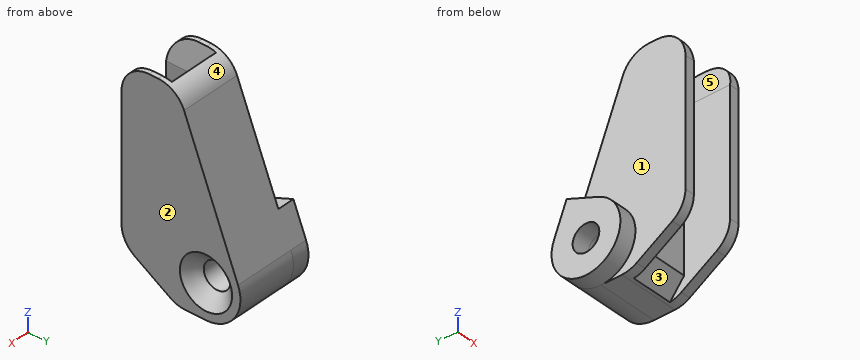
from build123d import *
from OCP.BRepFilletAPI import BRepFilletAPI_MakeChamfer

# Parameters (mm, degrees)
SKETCH1_R                                       = 2.2
BOSS_EXTRUDE1_DEPTH                             = 11
CUT_EXTRUDE1_REACH                              = 42.774
SKETCH2_W                                       = 7.5
SKETCH2_H                                       = 8.25
CHAMFER3_SIZE                                   = 5
CHAMFER3_SIZE2                                  = 0.881634904
FILLET1_R                                       = 5
CHAMFER1_SIZE                                   = 2.212207332
CHAMFER1_SIZE_2                                 = 4
CSK_FOR_M4_FLAT_HEAD_MACHINE_SCREW1_D           = 4.8
CSK_FOR_M4_FLAT_HEAD_MACHINE_SCREW1_CSINK_D     = 9.4
CSK_FOR_M4_FLAT_HEAD_MACHINE_SCREW1_CSINK_ANGLE = 90
BOSS_EXTRUDE2_START                             = 3.12
SKETCH6_R                                       = 2.4
BOSS_EXTRUDE2_DEPTH                             = 3.12


with BuildPart() as part:
    # Sketch1 → Boss-Extrude1 (new body)
    with BuildSketch(Plane(origin=(0, 0, 0), x_dir=(0, 0, -1), z_dir=(1, 0, 0))):
        with BuildLine():
            Line((-30, -15.2), (-30, -5.2))
            Line((-30, -5.2), (-2.280651189, 5.765295322))
            ThreePointArc((-2.280651189, 5.765295322), (3.485682331, 5.12737932), (6.2, 0))
            Line((6.2, 0), (6.2, -5.2))
            Line((6.2, -5.2), (0, -15.2))
            Line((0, -15.2), (-30, -15.2))
        make_face()
        Circle(SKETCH1_R, mode=Mode.SUBTRACT)
    extrude(amount=BOSS_EXTRUDE1_DEPTH)

    # Cut-Extrude1: up to this plane
    cut_extrude1_end = Plane(origin=(11, -5.2, -6.2), z_dir=(0, 0.5269396688616753, 0.8499026917123795))
    # Sketch2 → Cut-Extrude1 (cut, up to the surface)
    with BuildSketch(Plane.XY.offset(30), mode=Mode.PRIVATE) as cut_extrude1_sk1:
        with Locations((5.5, -11.075)):
            Rectangle(SKETCH2_W, SKETCH2_H)
    cut_extrude1_tool1 = split(extrude(cut_extrude1_sk1.sketch, amount=-CUT_EXTRUDE1_REACH, mode=Mode.PRIVATE), bisect_by=cut_extrude1_end, keep=Keep.BOTH, mode=Mode.PRIVATE)
    add(cut_extrude1_tool1.solids().sort_by_distance((5.5, -11.075, 30))[0], mode=Mode.SUBTRACT)

    # Chamfer3: one chamfer whose edges measure the first distance from different faces: ONE call of the kernel's chamfer builder (chamfer() names one face for all edges)
    chamfer3_edges_1 = [part.edges().sort_by_distance(p)[0] for p in [
        (1.75, -11.075, 30),
    ]]
    chamfer3_side_1 = [part.faces().sort_by_distance(p)[0] for p in [
        (1.75, -10.966989173, 13.687766644),
    ]]
    chamfer3_edges_2 = [part.edges().sort_by_distance(p)[0] for p in [
        (9.25, -11.075, 30),
    ]]
    chamfer3_side_2 = [part.faces().sort_by_distance(p)[0] for p in [
        (9.25, -10.966989173, 13.687766644),
    ]]
    chamfer3 = BRepFilletAPI_MakeChamfer(part.part.solid().wrapped)
    for e in chamfer3_edges_1:
        chamfer3.Add(CHAMFER3_SIZE, CHAMFER3_SIZE2, e.wrapped, chamfer3_side_1[0].wrapped)  # the first distance lies on this face
    for e in chamfer3_edges_2:
        chamfer3.Add(CHAMFER3_SIZE, CHAMFER3_SIZE2, e.wrapped, chamfer3_side_2[0].wrapped)  # the first distance lies on this face
    add(Compound.cast(chamfer3.Shape()), mode=Mode.REPLACE)

    # Fillet1
    # the kernel refuses this fillet: 5 mm, written as the material it takes off along each edge
    with BuildSketch(Plane(origin=(-12.5, -15.2, 30), x_dir=(0, 1, 0), z_dir=(1, 0, 0)), Plane(origin=(-2.368365096, -15.2, 30), x_dir=(0, 1, 0), z_dir=(1, 0, 0))) as fillet1_piece_1:
        with BuildLine():
            CenterArc((FILLET1_R, -FILLET1_R), FILLET1_R, 90, 90)
            Line((0, -FILLET1_R), (0, 0))
            Line((0, 0), (FILLET1_R, 0))
        make_face()
    extrude(amount=25.868365096, mode=Mode.SUBTRACT)
    with BuildSketch(Plane(origin=(-3.560590452, -5.2, -6.2), x_dir=(0, -0.8499026917123794, 0.5269396688616755), z_dir=(1, 0, 0))) as fillet1_piece_2:
        with BuildLine():
            CenterArc((FILLET1_R * 0.28484723614, -FILLET1_R), FILLET1_R, 90, 31.798912824)
            Line((-FILLET1_R * 0.242092432722, -FILLET1_R * 0.150097308288), (0, 0))
            Line((0, 0), (FILLET1_R * 0.28484723614, 0))
        make_face()
    extrude(amount=18.121180903, mode=Mode.SUBTRACT)
    with BuildSketch(Plane(origin=(-6.95756608, -15.2, 0), x_dir=(0, 0.8499026917123792, -0.5269396688616758), z_dir=(1, 0, 0)), Plane(origin=(2.29243392, -15.2, 0), x_dir=(0, 0.8499026917123792, -0.5269396688616758), z_dir=(1, 0, 0))) as fillet1_piece_3:
        with BuildLine():
            CenterArc((FILLET1_R * 0.556605286407, FILLET1_R), FILLET1_R, 211.798912824, 58.201087176)
            Line((-FILLET1_R * 0.293297405306, FILLET1_R * 0.473060331138), (0, 0))
            Line((0, 0), (FILLET1_R * 0.556605286407, 0))
        make_face()
    extrude(amount=15.66513216, mode=Mode.SUBTRACT)
    with BuildSketch(Plane(origin=(-8.497719093, -5.2, 30), x_dir=(0, -1, 0), z_dir=(1, 0, 0))) as fillet1_piece_4:
        with BuildLine():
            CenterArc((FILLET1_R * 0.679817527413, FILLET1_R), FILLET1_R, 201.582895238, 68.417104762)
            Line((-FILLET1_R * 0.250068814892, FILLET1_R * 0.632153034001), (0, 0))
            Line((0, 0), (FILLET1_R * 0.679817527413, 0))
        make_face()
    extrude(amount=27.995438185, mode=Mode.SUBTRACT)

    # Chamfer1
    # the kernel refuses this chamfer: 4, 2.212207332 mm, written as the material it takes off along each edge
    with BuildSketch(Plane(origin=(1.75, -6.95, -5.115), x_dir=(0, -0.04228471314336273, 0.9991056015428917), z_dir=(1, 0, 0))) as chamfer1_piece_1:
        Polygon((CHAMFER1_SIZE * 0.999105601467, -CHAMFER1_SIZE * 0.0422847131402), (-CHAMFER1_SIZE_2 * 0.562406266354, -CHAMFER1_SIZE_2 * 0.826861047315), (0, 0), align=None)
    extrude(amount=7.5, mode=Mode.SUBTRACT)

    # CSK for M4 Flat Head Machine Screw1 (through all)
    with Locations(Plane(origin=(11, 0, 0), x_dir=(0, 0, -1), z_dir=(1, 0, 0))):
        with Locations((0, 0)):
            CounterSinkHole(CSK_FOR_M4_FLAT_HEAD_MACHINE_SCREW1_D / 2, CSK_FOR_M4_FLAT_HEAD_MACHINE_SCREW1_CSINK_D / 2, counter_sink_angle=CSK_FOR_M4_FLAT_HEAD_MACHINE_SCREW1_CSINK_ANGLE)

    # Sketch6 → Boss-Extrude2 (add)
    with BuildSketch(Plane.ZY.offset(BOSS_EXTRUDE2_START)):
        with BuildLine():
            Line((8.045946511, 3.484644133), (5.765295322, -2.280651189))
            ThreePointArc((5.765295322, -2.280651189), (-5.689343339, -2.464015497), (2.280651189, 5.765295322))
            Line((2.280651189, 5.765295322), (8.045946511, 3.484644133))
        make_face()
        with Locations(Location((0, 0, 0), (0, 0, 180))):
            Circle(SKETCH6_R, mode=Mode.SUBTRACT)
    extrude(amount=-BOSS_EXTRUDE2_DEPTH)


solid = part.part
Here's how the part is built. I have some questions about the finished solid (model axes, mm). Face numbers are marked on the shaded views. A direction names the side the tool comes from. Give positions to 0.01 mm unless a question says otherwise; leave off trailing zeros. Order: outer loops, then holes, each group sorted by start corner. A loop starts at its lowest first (then second) coordinate and runs counter-clockwise, first axis right, second up. Notation, with made-up numbers: (58.5, -15.75) -> (64.5, -15.75) arc R17 cw to (64.5, -9.75) -> close; hole circle Ø9 at (70, 72). An arc over 180 degrees is marked (long way). One line per item, written item: value. Start each with the question number.
1. Imagine slicing it at B-B, the plane z = 0. List the corners of the cut face in (x, y) for me, plus the area to 3 significant figures.
2. We'd pull the mould along X, two halves only. Please class the marked faces 1, 2 and 3: released by +X, released by -X, zero draft, split by the parting line, or undercut.
3. Imagine slicing it at A-A, the plane x = 2.75. List the corners of the cut face in (y, z) for me.
4. Imagine slicing it at C-C, the plane y = -11.5. List the corners of the cut face in (x, z) for me, plus the area to 3 significant figures.
5. I need wall thicknesses on probe 1 along Y at (x, z) = (7.25, 0); probe 2 along X at (y, z) = (-8.75, 16); probe 3 along Y at (x, z) = (-0.6, 0). Which ranges of each line are inside material? Lowest first, please. Write a range as from..to.
6. Imagine slicing it at D-D, the plane z = 27.5. List the corners of the cut face in (x, y) for me, plus the area to 3 significant figures.
7. For the marked faces 4 and 5, which set-ups out of +Z, -Z, +X, -X, +Y, -Y let a thin tool reach every point of the face, with its end or its side?
8. Will these pins go through, and if not, where does the flat tip stop? pin 1 Ø1 at (x, y) = (6, -5) entering from -Z; pin 2 Ø1 at (y, z) = (-10.5, 19.5) entering from -X; pin 3 Ø10 at (y, z) = (-7.5, 7) entering from -X; pin 4 Ø4.5 at (x, z) = (4.5, 17) entering from -Y.
Values follow:
1. outline: (-3.12, -6.2) -> (0, -6.2) -> (0, -14.35) -> (1.75, -14.35) -> (1.75, -6.95) -> (9.25, -6.95) -> (9.25, -14.35) -> (11, -14.35) -> (11, -4.7) -> (8.7, -2.4) -> (-3.12, -2.4) -> close; (-3.12, 2.4) -> (8.7, 2.4) -> (11, 4.7) -> (11, 6.2) -> (-3.12, 6.2) -> close
1. area: 136 mm2
2. face 1: released by -X
2. face 2: released by +X
2. face 3: undercut
3. outline: (-6.95, -2.9) -> (-4.38, -6.16) arc R5 ccw to (-3.78, -6.2) -> (0, -6.2) arc R6.2 ccw to (5.77, 2.28) -> (-3.95, 26.84) arc R5 ccw to (-6.95, 29.72) -> close; hole circle Ø4.8 at (0, 0)
4. outline: (0, -2.29) -> (1.75, -2.29) -> (1.75, 25) -> (0.9, 29.83) -> (0, 29.83) -> close; (9.25, -2.29) -> (11, -2.29) -> (11, 29.83) -> (10.1, 29.83) -> (9.25, 25) -> close
4. area: 108 mm2
5. probe 1: y = -6.95..-2.4, 2.4..6.2
5. probe 2: x = 0..1.75, 9.25..11
5. probe 3: y = -6.2..-2.4, 2.4..6.2
6. outline: (0, -14.53) -> (1.31, -14.53) -> (1.31, -6.95) -> (9.69, -6.95) -> (9.69, -14.53) -> (11, -14.53) -> (11, -4.27) -> (0, -4.27) -> close
6. area: 49.3 mm2
7. face 4: +Z, +X, -X, +Y
7. face 5: +Z, -Y
8. pin 1: stops at z = -6.02
8. pin 2: stops at x = 0
8. pin 3: stops at x = -3.12
8. pin 4: stops at y = -6.95
